Geometry: final body of the model. Coordinates: model frame, mm. A direction names the side the tool comes from. Give positions to 0.01 mm unless a question says otherwise; leave off trailing zeros. Order: outer loops, then holes, each group sorted by start corner. A loop starts at its lowest first (then second) coordinate and runs counter-clockwise, first axis right, second up. Notation, with made-up numbers: (-14, 78) -> (41, 78) arc R21 ccw to (41, 100) -> close; hole circle Ø7 at (50.5, -26.75). An arc over 180 degrees is marked (long way). Write item = value, one per line.
```python
from build123d import *

# Parameters (mm, degrees)
BOSS_EXTRUDE1_DEPTH      = 6.35
SKETCH2_R                = 3.175
SKETCH2_R_2              = 1.27
BOSS_EXTRUDE2_DEPTH      = 32.213991
BOSS_EXTRUDE2_DEPTH_BACK = 26.506426
CUT_EXTRUDE1_START       = 32.213991
SKETCH2_7_R              = 3.175
SKETCH2_7_R_2            = 1.27
CUT_EXTRUDE1_DEPTH       = 19.05
CUT_EXTRUDE2_START       = -26.506426
SKETCH2_8_R              = 3.175
SKETCH2_8_R_2            = 1.27
CUT_EXTRUDE2_DEPTH       = 19.05
BOSS_EXTRUDE3_DEPTH      = 19.05
BOSS_EXTRUDE3_DEPTH_BACK = 24.13
CUT_EXTRUDE3_DEPTH       = 19.05
CUT_EXTRUDE4_START       = 3.81
SKETCH6_R                = 3.175
SKETCH6_R_2              = 1.27
CUT_EXTRUDE4_DEPTH       = 16.51
SKETCH6_4_R              = 1.27
CUT_EXTRUDE5_DEPTH       = 22.86


with BuildPart() as part:
    # Sketch1 → Boss-Extrude1 (new body)
    with BuildSketch(Plane(origin=(0, 0, 0), x_dir=(1, 0, 0), z_dir=(0, 1, 0))):
        Polygon((-26.506426074, 19.099553328), (32.213990648, 19.099553328), (9.353990648, 41.959553328), (-23.666009352, 41.959553328), align=None)
    extrude(amount=BOSS_EXTRUDE1_DEPTH)

    # Sketch2 → Boss-Extrude2 (add, two sides)
    with BuildSketch(Plane(origin=(0, 0, 0), x_dir=(0, 0, -1), z_dir=(1, 0, 0))) as boss_extrude2_sk:
        with BuildLine():
            ThreePointArc((19.099553328, 3.175), (18.169617358, 0.92993597), (15.924553328, 0))
            Line((15.924553328, 0), (19.099553328, 0))
            Line((19.099553328, 0), (19.099553328, 3.175))
        make_face()
        with BuildLine():
            ThreePointArc((15.924553328, 6.35), (18.169617358, 5.42006403), (19.099553328, 3.175))
            Line((19.099553328, 3.175), (19.099553328, 6.35))
            Line((19.099553328, 6.35), (15.924553328, 6.35))
        make_face()
        with Locations((15.924553328, 3.175)):
            Circle(SKETCH2_R)
        with Locations((15.924553328, 3.175)):
            Circle(SKETCH2_R_2, mode=Mode.SUBTRACT)
        with BuildLine():
            Line((12.749553328, 3.175), (12.749553328, 0))
            Line((12.749553328, 0), (15.924553328, 0))
            ThreePointArc((15.924553328, 0), (13.679489298, 0.92993597), (12.749553328, 3.175))
        make_face()
    extrude(amount=BOSS_EXTRUDE2_DEPTH)
    extrude(boss_extrude2_sk.sketch, amount=-BOSS_EXTRUDE2_DEPTH_BACK)

    # Sketch2<7> → Cut-Extrude1 (cut)
    with BuildSketch(Plane(origin=(0, 0, 0), x_dir=(0, 0, -1), z_dir=(1, 0, 0)).offset(CUT_EXTRUDE1_START)):
        with Locations((15.924553328, 3.175)):
            Circle(SKETCH2_7_R)
        with Locations((15.924553328, 3.175)):
            Circle(SKETCH2_7_R_2, mode=Mode.SUBTRACT)
        with BuildLine():
            ThreePointArc((19.099553328, 3.175), (18.169617358, 0.92993597), (15.924553328, 0))
            Line((15.924553328, 0), (19.099553328, 0))
            Line((19.099553328, 0), (19.099553328, 3.175))
        make_face()
        with BuildLine():
            Line((12.749553328, 3.175), (12.749553328, 0))
            Line((12.749553328, 0), (15.924553328, 0))
            ThreePointArc((15.924553328, 0), (13.679489298, 0.92993597), (12.749553328, 3.175))
        make_face()
        with BuildLine():
            ThreePointArc((15.924553328, 6.35), (18.169617358, 5.42006403), (19.099553328, 3.175))
            Line((19.099553328, 3.175), (19.099553328, 6.35))
            Line((19.099553328, 6.35), (15.924553328, 6.35))
        make_face()
    extrude(amount=-CUT_EXTRUDE1_DEPTH, mode=Mode.SUBTRACT)

    # Sketch2<8> → Cut-Extrude2 (cut)
    with BuildSketch(Plane(origin=(0, 0, 0), x_dir=(0, 0, -1), z_dir=(1, 0, 0)).offset(CUT_EXTRUDE2_START)):
        with Locations((15.924553328, 3.175)):
            Circle(SKETCH2_8_R)
        with Locations((15.924553328, 3.175)):
            Circle(SKETCH2_8_R_2, mode=Mode.SUBTRACT)
        with BuildLine():
            ThreePointArc((19.099553328, 3.175), (18.169617358, 0.92993597), (15.924553328, 0))
            Line((15.924553328, 0), (19.099553328, 0))
            Line((19.099553328, 0), (19.099553328, 3.175))
        make_face()
        with BuildLine():
            Line((12.749553328, 3.175), (12.749553328, 0))
            Line((12.749553328, 0), (15.924553328, 0))
            ThreePointArc((15.924553328, 0), (13.679489298, 0.92993597), (12.749553328, 3.175))
        make_face()
        with BuildLine():
            ThreePointArc((15.924553328, 6.35), (18.169617358, 5.42006403), (19.099553328, 3.175))
            Line((19.099553328, 3.175), (19.099553328, 6.35))
            Line((19.099553328, 6.35), (15.924553328, 6.35))
        make_face()
    extrude(amount=CUT_EXTRUDE2_DEPTH, mode=Mode.SUBTRACT)

    # Sketch5 → Boss-Extrude3 (add, two sides)
    with BuildSketch(Plane(origin=(0, 0, 0), x_dir=(0, 0, -1), z_dir=(1, 0, 0))) as boss_extrude3_sk:
        with BuildLine():
            Line((48.309553328, 0), (48.309553328, 3.175))
            ThreePointArc((48.309553328, 3.175), (47.379617358, 5.42006403), (45.134553328, 6.35))
            Line((45.134553328, 6.35), (41.959553328, 6.35))
            Line((41.959553328, 6.35), (41.959553328, 0))
            Line((41.959553328, 0), (48.309553328, 0))
        make_face()
    extrude(amount=BOSS_EXTRUDE3_DEPTH)
    extrude(boss_extrude3_sk.sketch, amount=-BOSS_EXTRUDE3_DEPTH_BACK)

    # Sketch3 → Cut-Extrude3 (cut)
    with BuildSketch(Plane(origin=(0, 6.35, 0), x_dir=(1, 0, 0), z_dir=(0, 1, 0))):
        Polygon((-23.666009352, 41.959553328), (-20.016630387, 71.330174364), (9.353990648, 41.959553328), (25.531438474, 33.85540027), (42.679810996, 71.330174364), (-40.952906467, 76.015398382), (-46.546209233, 30.999855332), align=None)
    extrude(amount=-CUT_EXTRUDE3_DEPTH, mode=Mode.SUBTRACT)

    # Sketch6 → Cut-Extrude4 (cut)
    with BuildSketch(Plane(origin=(3.003990648, 0, 0), x_dir=(0, 1, 0), z_dir=(-1, 0, 0)).offset(CUT_EXTRUDE4_START)):
        with Locations((3.175, 45.134553328)):
            Circle(SKETCH6_R)
        with Locations(Location((3.175, 45.134553328, 0), (0, 0, 270))):
            Circle(SKETCH6_R_2, mode=Mode.SUBTRACT)
        with BuildLine():
            ThreePointArc((3.175, 48.309553328), (5.42006403, 47.379617358), (6.35, 45.134553328))
            Line((6.35, 45.134553328), (6.35, 48.309553328))
            Line((6.35, 48.309553328), (3.175, 48.309553328))
        make_face()
        with BuildLine():
            Line((0, 48.309553328), (0, 45.134553328))
            ThreePointArc((0, 45.134553328), (0.92993597, 47.379617358), (3.175, 48.309553328))
            Line((3.175, 48.309553328), (0, 48.309553328))
        make_face()
        with BuildLine():
            Line((3.175, 41.959553328), (6.35, 41.959553328))
            Line((6.35, 41.959553328), (6.35, 45.134553328))
            ThreePointArc((6.35, 45.134553328), (5.42006403, 42.889489298), (3.175, 41.959553328))
        make_face()
        with BuildLine():
            Line((0, 41.959553328), (3.175, 41.959553328))
            ThreePointArc((3.175, 41.959553328), (0.92993597, 42.889489298), (0, 45.134553328))
            Line((0, 45.134553328), (0, 41.959553328))
        make_face()
    extrude(amount=CUT_EXTRUDE4_DEPTH, mode=Mode.SUBTRACT)

    # Sketch6<4> → Cut-Extrude5 (cut)
    with BuildSketch(Plane(origin=(3.003990648, 0, 0), x_dir=(0, 1, 0), z_dir=(-1, 0, 0))):
        with Locations(Location((3.175, 45.134553328, 0), (0, 0, 270))):
            Circle(SKETCH6_4_R)
    extrude(amount=CUT_EXTRUDE5_DEPTH, mode=Mode.SUBTRACT)


solid = part.part
```
1) Reachability of faces 5 (the face through (13.164, 2.5, -17.3)), 6 (the face through (-3, 6.35, -31)), 7 (the face through (-9, 3, -41.96)), 8 (the face through (1.126, 3.231, -46.403)), 9 (the face through (-7.456, 2.5, -17.3)) from +Z, -Z, +X, -X, +Y, -Y: full face, straight path, thin tool, end or side. Return the list, or none.
Check sheet entries:
face_5 = +Z, +X, +Y, -Y
face_6 = +Z, -Z, +X, -X, +Y
face_7 = -Z, +Y, -Y
face_8 = none
face_9 = +Z, -X, +Y, -Y
2) Section query A-A (x = 2). Output: boundary loops of the cut face in (y, z) (3 decimals), plus the area to 3 significant figures.
Check sheet entries:
outline = (0, -48.31) -> (3.175, -48.31) arc R3.175 ccw to (6.35, -45.135) -> (6.35, -15.925) arc R3.175 ccw to (3.175, -12.75) -> (0, -12.75) -> close; hole circle Ø2.54 at (3.175, -45.135); hole circle Ø2.54 at (3.175, -15.925)
area = 211 mm²
3) Mould query, pull axis Y, two halves, no side actions, for faces 1 (the face through (-20, 2, -48.31)), 2 (the face through (-18.568, 3.231, -46.403)), 3 (the face through (3, 5.44, -13.7)), 4 (the face through (2.998, 4.246, -16.607)). Classes: +Y half, -Y half, draft (parallel to the pull), parting line (faces both ways), or undercut.
Check sheet entries:
face_1 = draft
face_2 = undercut
face_3 = +Y half
face_4 = undercut
4) First-contact query: P1, Ø2, axis at y = 3.18, z = -45.13, coming from the -X side; P2, Ø3, axis at y = 3, z = -15, coming from the +X side; P3, Ø1, axis at x = -20.5, y = 2, coming from the +Z side; P4, Ø2, axis at y = 3.18, z = -15.92, coming from the -X side. Flat tips, straight axial feed; report the tip coordinate or a pass-through.
Check sheet entries:
P1 = -23.4
P2 = 13.16
P3 = -19.1
P4 = through
5) Section query D-D (x = -12). Output: boundary loops of the cut face in (y, z).
Check sheet entries:
outline = (0, -41.96) -> (6.35, -41.96) -> (6.35, -19.1) -> (0, -19.1) -> close
6) Line query: line 1 (X direction, y = 4, z = -14.5); line 2 (Z direction, x = 0, y = 4.25); line 3 (Z direction, x = -16.5, y = 4.5). Output: solid intervals per line, ascending. Write a range as from..to.
Check sheet entries:
line_1 = -7.46..13.16
line_2 = -48.12..-45.81, -44.46..-16.6, -15.25..-12.94
line_3 = -41.96..-19.1
7) Section query B-B (y = 3.75). Output: boundary loops of the cut face in (x, z), plus the area to 3 significant figures.
Check sheet entries:
outline = (-26.51, -19.1) -> (-22.88, -48.26) -> (-17.32, -48.26) -> (-17.32, -46.27) -> (-19.86, -46.27) -> (-19.86, -44) -> (-17.32, -44) -> (-17.32, -41.96) -> (-0.81, -41.96) -> (-0.81, -44) -> (3, -44) -> (3, -46.27) -> (-0.81, -46.27) -> (-0.81, -48.26) -> (3.06, -48.26) -> (32.21, -19.1) -> (13.16, -19.1) -> (13.16, -17.06) -> (-7.46, -17.06) -> (-7.46, -19.1) -> close; (-7.46, -14.79) -> (13.16, -14.79) -> (13.16, -12.8) -> (-7.46, -12.8) -> close
area = 1,200 mm²
8) Section query C-C (z = -20.5). Output: boundary loops of the cut face in (x, y), plus the area to 3 significant figures.
Check sheet entries:
outline = (-26.33, 0) -> (30.81, 0) -> (30.81, 6.35) -> (-26.33, 6.35) -> close
area = 363 mm²
